from build123d import *

# Parameters (mm, degrees)
BOSS_EXTRUDE1_DEPTH = 5.87
SKETCH6_R           = 0.75
BOSS_EXTRUDE2_DEPTH = 10.25
FILLET1_R           = 0.1
FILLET2_R           = 1.4
FILLET3_R           = 1.4


with BuildPart() as part:
    # Sketch1 → Boss-Extrude1 (new, symmetric)
    with BuildSketch(Plane.XY):
        Polygon((-9.25, 0), (9.25, 0), (9.25, 3), (5.5, 6), (-5.5, 6), (-9.25, 3), align=None)
    extrude(amount=BOSS_EXTRUDE1_DEPTH, both=True)

    # Sketch2 → Revolve5 (revolve)
    with BuildSketch(Plane.XY, mode=Mode.PRIVATE) as revolve5_sk:
        with BuildLine():
            ThreePointArc((3.5, 9), (3.465409062, 7.321803021), (4.5, 6))
            Line((4.5, 6), (0, 6))
            Line((0, 6), (0, 13.5))
            Line((0, 13.5), (4.5, 13.5))
            Line((4.5, 13.5), (4.5, 13.7))
            Line((4.5, 13.7), (5, 13.7))
            Line((5, 13.7), (5, 11))
            Line((5, 11), (3.5, 11))
            Line((3.5, 11), (3.5, 9))
        make_face()
    revolve(revolve5_sk.sketch.rotate(Axis((0, 13.5, 0), (0, -1, 0)), 90), axis=Axis((0, 13.5, 0), (0, -1, 0)))

    # Sketch3 → Revolve6 (revolve)
    with BuildSketch(Plane.XY, mode=Mode.PRIVATE) as revolve6_sk:
        with BuildLine():
            Line((0, 13.5), (0, 14.541750876))
            ThreePointArc((0, 14.541750876), (2.431447351, 14.278254553), (4.75, 13.5))
            Line((4.75, 13.5), (0, 13.5))
        make_face()
    revolve(revolve6_sk.sketch.rotate(Axis((0, 20.298095722, 0), (0, -1, 0)), 90), axis=Axis((0, 20.298095722, 0), (0, -1, 0)))

    # Sketch6 → Boss-Extrude2 (add, symmetric)
    with BuildSketch(Plane.ZY):
        with Locations((3.87, 1.5)):
            Circle(SKETCH6_R)
    extrude(amount=BOSS_EXTRUDE2_DEPTH, both=True)

    # Fillet1
    # the kernel refuses this fillet: 0.1 mm, written as the material it takes off along each edge
    with BuildSketch(Plane(origin=(0, 11, 0), x_dir=(0, 0, 1), z_dir=(1, 0, 0))) as fillet1_piece_1:
        with BuildLine():
            CenterArc((5 - FILLET1_R, -FILLET1_R), FILLET1_R, 0, 90)
            Line((5, -FILLET1_R), (5, 0))
            Line((5, 0), (5 - FILLET1_R, 0))
        make_face()
    revolve(axis=Axis((0, 11, 0), (0, -1, 0)), mode=Mode.SUBTRACT)
    with BuildSketch(Plane(origin=(0, 13.7, 0), x_dir=(0, 0, 1), z_dir=(1, 0, 0))) as fillet1_piece_2:
        with BuildLine():
            CenterArc((5 - FILLET1_R, FILLET1_R), FILLET1_R, 270, 90)
            Line((5 - FILLET1_R, 0), (5, 0))
            Line((5, 0), (5, FILLET1_R))
        make_face()
    revolve(axis=Axis((0, 13.7, 0), (0, -1, 0)), mode=Mode.SUBTRACT)
    with BuildSketch(Plane(origin=(0, 13.7, 0), x_dir=(0, 0, 1), z_dir=(1, 0, 0))) as fillet1_piece_3:
        with BuildLine():
            CenterArc((4.59932915, 0.1), FILLET1_R, 186.640387385, 83.359612615)
            Line((4.5, 0.088436266), (4.5, 0))
            Line((4.5, 0), (4.59932915, 0))
        make_face()
    revolve(axis=Axis((0, 13.7, 0), (0, -1, 0)), mode=Mode.SUBTRACT)

    # Fillet2
    fillet2_edges = [part.edges().sort_by_distance(p)[0] for p in [
        (-9.25, 3, 0),
        (-5.5, 6, 0),
        (9.25, 3, 0),
        (0, 0, -5.87),
    ]]
    fillet(fillet2_edges, radius=FILLET2_R)

    # Fillet3
    fillet3_edges = [part.edges().sort_by_distance(p)[0] for p in [
        (5.5, 6, 0),
    ]]
    fillet(fillet3_edges, radius=FILLET3_R)


solid = part.part
Here's how the part is built. I have some questions about the finished solid (model axes, mm). A direction names the side the tool comes from. Round coordinates to 2 decimals unless told otherwise and drop trailing zeros. Loops run counter-clockwise (first coordinate to the right, second up) from the corner with the lowest first, then second, coordinate; pieces in that order, holes last.
1. If we section it at B-B on x = 0: Write out the boundary of the cut face in (y, z), plus the area to 3 significant figures.
Answer list:
outline: (0, -4.47) arc R1.4 ccw to (1.4, -5.87) - (6, -5.87) - (6, -4.5) arc R2.5 cw to (9, -3.5) - (11, -3.5) - (11, -4.9) arc R0.1 ccw to (11.1, -5) - (13.6, -5) arc R0.1 ccw to (13.7, -4.9) - (13.7, -4.6) arc R0.1 ccw to (13.61, -4.5) arc R11.35 ccw to (13.61, 4.5) arc R0.1 ccw to (13.7, 4.6) - (13.7, 4.9) arc R0.1 ccw to (13.6, 5) - (11.1, 5) arc R0.1 ccw to (11, 4.9) - (11, 3.5) - (9, 3.5) arc R2.5 cw to (6, 4.5) - (6, 5.87) - (0, 5.87) - close
area: 137 mm2
2. We'd pull the mould along Y, two halves only. Please class faces 4 (the face through (9.743, 1.044, 3.275)), 5 (the face through (9.25, 1, 0)), 6 (the face through (4.5, 6, 1.4)): +Y half, -Y half, draft (parallel to the pull), parting line (faces both ways), or undercut.
Answer list:
face 4: parting line
face 5: draft
face 6: undercut
3. For P1, Ø5, axis at x = -5, z = 4.5, coming from the +Y side; P2, Ø3, axis at x = 0.5, z = 2.5, coming from the +Y side; P3, Ø1.5, axis at y = 11.5, z = 4, coming from the -X side, each with a flat end and sliding along its axis, tell me the tip position at first contact or that it passes through.
Answer list:
P1: stops at y = 13.73
P2: stops at y = 14.49
P3: stops at x = -3.8
4. If I drill on line 1 along Y through (x, z) = (3, 5); line 2 along Y through (x, z) = (9, 4.75); line 3 along X through (y, z) = (1, 0.75), over which ranges is the centre line in solid material (lowest first)?
Answer list:
line 1: y = 0 to 6
line 2: y = 0 to 3.13
line 3: x = -9.25 to 9.25
5. If we section it at C-C on y = 12: Write out the boundary of the cut face in (x, z).
Answer list:
outline: circle Ø10 at (0, 0)
6. If we section it at A-A on z = 0: Write out the boundary of the cut face in (x, y).
Answer list:
outline: (-9.25, 0) - (9.25, 0) - (9.25, 2.33) arc R1.4 ccw to (8.72, 3.42) - (5.88, 5.69) arc R1.4 ccw to (5.01, 6) - (4.5, 6) arc R2.5 cw to (3.5, 9) - (3.5, 11) - (4.9, 11) arc R0.1 ccw to (5, 11.1) - (5, 13.6) arc R0.1 ccw to (4.9, 13.7) - (4.6, 13.7) arc R0.1 ccw to (4.5, 13.61) arc R11.35 ccw to (-4.5, 13.61) arc R0.1 ccw to (-4.6, 13.7) - (-4.9, 13.7) arc R0.1 ccw to (-5, 13.6) - (-5, 11.1) arc R0.1 ccw to (-4.9, 11) - (-3.5, 11) - (-3.5, 9) arc R2.5 cw to (-4.5, 6) - (-5.01, 6) arc R1.4 ccw to (-5.88, 5.69) - (-8.72, 3.42) arc R1.4 ccw to (-9.25, 2.33) - close
7. Which directions (+Z, -Z, +X, -X, +Y, -Y) give clear straight access to the entire face, cutting with the end or side of a thin tool? Please do faces 1 (the face through (-9.757, 1.044, 3.275)), 2 (the face through (3.2, 11, 2.1)), 3 (the face through (0, 0, 1)).
Answer list:
face 1: -X
face 2: none
face 3: +Z, -Z, +X, -X, -Y
8. If we section it at D-D on z = 5.25: Write out the boundary of the cut face in (x, y), plus the area to 3 significant figures.
Answer list:
outline: (-9.25, 0) - (9.25, 0) - (9.25, 2.33) arc R1.4 ccw to (8.72, 3.42) - (5.88, 5.69) arc R1.4 ccw to (5.01, 6) - (-5.01, 6) arc R1.4 ccw to (-5.88, 5.69) - (-8.72, 3.42) arc R1.4 ccw to (-9.25, 2.33) - close
area: 99.6 mm2
